from build123d import *

# Parameters (mm, degrees)
SKETCH_W        = 50
SKETCH_H        = 52
PAD_DEPTH       = 1
SKETCH001_W     = 3
SKETCH001_H     = 3
PAD001_DEPTH    = 4
FILLET_R        = 1
FILLET001_R     = 1
FILLET002_R     = 1
FILLET003_R     = 1
SKETCH002_R     = 2.75
POCKET_DEPTH    = 1
SKETCH003_W     = 2
SKETCH003_H     = 7
POCKET001_DEPTH = 1
FILLET004_R     = 0.5
SKETCH004_R     = 3.8
PAD002_DEPTH    = 2
SKETCH005_R     = 2.8
POCKET002_DEPTH = 2
SKETCH006_W     = 8
SKETCH006_H     = 36
POCKET003_DEPTH = 1
SKETCH007_W     = 6
SKETCH007_H     = 36
POCKET004_DEPTH = 1


with BuildPart() as part:
    # Sketch → Pad (new body)
    with BuildSketch(Plane.XY):
        Rectangle(SKETCH_W, SKETCH_H)
    extrude(amount=PAD_DEPTH)

    # Sketch001 (on Face6 of Pad) → Pad001 (join)
    with BuildSketch(Plane.XY.offset(1)):
        with Locations((-22.5, 23.5)):
            Rectangle(SKETCH001_W, SKETCH001_H)
        with Locations((22.5, 23.5)):
            Rectangle(SKETCH001_W, SKETCH001_H)
        with Locations((-22.5, -23.5)):
            Rectangle(SKETCH001_W, SKETCH001_H)
        with Locations((22.5, -23.5)):
            Rectangle(SKETCH001_W, SKETCH001_H)
    extrude(amount=PAD001_DEPTH)

    # Fillet
    fillet_edges = [part.edges().sort_by_distance(p)[0] for p in [
        (-25, -26, 0.5),
    ]]
    fillet(fillet_edges, radius=FILLET_R)

    # Fillet001
    fillet001_edges = [part.edges().sort_by_distance(p)[0] for p in [
        (25, -26, 0.5),
    ]]
    fillet(fillet001_edges, radius=FILLET001_R)

    # Fillet002
    fillet002_edges = [part.edges().sort_by_distance(p)[0] for p in [
        (-25, 26, 0.5),
    ]]
    fillet(fillet002_edges, radius=FILLET002_R)

    # Fillet003
    fillet003_edges = [part.edges().sort_by_distance(p)[0] for p in [
        (25, 26, 0.5),
    ]]
    fillet(fillet003_edges, radius=FILLET003_R)

    # Sketch002 (on Face1 of Fillet003) → Pocket (cut)
    with BuildSketch(Plane(origin=(0, 0, 0), x_dir=(1, 0, 0), z_dir=(0, 0, -1))):
        with Locations((-8, 20.5)):
            Circle(SKETCH002_R)
    extrude(amount=-POCKET_DEPTH, mode=Mode.SUBTRACT)

    # Sketch003 (on Face11 of Pocket) → Pocket001 (cut)
    with BuildSketch(Plane.XY.offset(1)):
        with Locations((15, -14.5)):
            Rectangle(SKETCH003_W, SKETCH003_H)
        with Locations((15, -5.5)):
            Rectangle(SKETCH003_W, SKETCH003_H)
        with Locations((11, -5.5)):
            Rectangle(SKETCH003_W, SKETCH003_H)
        with Locations((11, -14.5)):
            Rectangle(SKETCH003_W, SKETCH003_H)
        with Locations((7, -5.5)):
            Rectangle(SKETCH003_W, SKETCH003_H)
        with Locations((7, -14.5)):
            Rectangle(SKETCH003_W, SKETCH003_H)
        with Locations((3, -5.5)):
            Rectangle(SKETCH003_W, SKETCH003_H)
        with Locations((3, -14.5)):
            Rectangle(SKETCH003_W, SKETCH003_H)
    extrude(amount=-POCKET001_DEPTH, mode=Mode.SUBTRACT)

    # Fillet004
    fillet004_edges = [part.edges().sort_by_distance(p)[0] for p in [
        (0, -26, 0),
        (25, 0, 0),
        (-25, 0, 0),
        (0, 26, 0),
    ]]
    fillet(fillet004_edges, radius=FILLET004_R)

    # Sketch004 (on Face51 of Fillet004) → Pad002 (join)
    with BuildSketch(Plane.XY.offset(1)):
        with Locations((-8, -20.5)):
            Circle(SKETCH004_R)
    extrude(amount=PAD002_DEPTH)

    # Sketch005 (on Face71 of Pad002) → Pocket002 (cut)
    with BuildSketch(Plane.XY.offset(3)):
        with Locations((-8, -20.5)):
            Circle(SKETCH005_R)
    extrude(amount=-POCKET002_DEPTH, mode=Mode.SUBTRACT)

    # Sketch006 (on Face51 of Pocket002) → Pocket003 (cut)
    with BuildSketch(Plane.XY.offset(1)):
        with Locations((-21, 0)):
            Rectangle(SKETCH006_W, SKETCH006_H)
    extrude(amount=-POCKET003_DEPTH, mode=Mode.SUBTRACT)

    # Sketch007 (on Face53 of Pocket003) → Pocket004 (cut)
    with BuildSketch(Plane.XY.offset(1)):
        with Locations((22, 0)):
            Rectangle(SKETCH007_W, SKETCH007_H)
    extrude(amount=-POCKET004_DEPTH, mode=Mode.SUBTRACT)


solid = part.part
Can you work these out from the model? Positions are in its coordinate system, mm. A direction names the side the tool comes from. Coordinates: 2 decimals unless noted, no trailing zeros. Order: outer loops, then holes, each group sorted by start corner. A loop starts at its lowest first (then second) coordinate and runs counter-clockwise, first axis right, second up. Notation, with made-up numbers: M -31,4.5 L 5,4.5 A22 cw 5,32.5 Z; hole C -23.75,76.25 d7. An arc over 180 degrees is marked long. Answer as CSV lines item,"result".
(1) I'm going to push flat-ended pins straight in: pin 1 (1.5 mm diameter, centred on x = -22, z = 2.5, fed in from +Y); pin 2 (0.9 mm diameter, centred on x = -23, z = 3.5, fed in from -Y); pin 3 (6.5 mm diameter, centred on x = -8, y = -20.5, fed in from +Z). Where does each tip first touch, or does it pass through?
Geometry check:
pin 1,"y = 25"
pin 2,"y = -25"
pin 3,"z = 3"
(2) Suppose I cut it at B-B on y = -4. Please give me the cut outline in (x, z), plus the area to 3 significant figures.
Geometry check:
outline,"M -17,0 L 2,0 L 2,1 L -17,1 Z; M 4,0 L 6,0 L 6,1 L 4,1 Z; M 8,0 L 10,0 L 10,1 L 8,1 Z; M 12,0 L 14,0 L 14,1 L 12,1 Z; M 16,0 L 19,0 L 19,1 L 16,1 Z"
area,"28.0 mm^2"
(3) If we mould it in two halves opening along Y, with no side actions, what happens to faces 1 (the flat face through (21, -24, 3)), 2 (the cylindrical face through (-5.414, -21.572, 2.014)), 3 (the flat face through (22, -25, 3))? For each: released by +Y, released by -Y, zero draft, split by the parting line, or undercut.
Geometry check:
face 1,"zero draft"
face 2,"undercut"
face 3,"released by -Y"
(4) Suppose I cut it at A-A on x = -8. Please give me the cut outline in (y, z).
Geometry check:
outline,"M -26,0.5 A0.5 ccw -25.5,0 L -23.25,0 L -23.25,1 L -23.3,1 L -23.3,3 L -24.3,3 L -24.3,1 L -26,1 Z; M -17.75,0 L 25.5,0 A0.5 ccw 26,0.5 L 26,1 L -16.7,1 L -16.7,3 L -17.7,3 L -17.7,1 L -17.75,1 Z"
(5) Suppose I cut it at D-D on y = 19. Please give me the cut outline in (x, z).
Geometry check:
outline,"M -25,0.5 A0.5 ccw -24.5,0 L 24.5,0 A0.5 ccw 25,0.5 L 25,1 L -25,1 Z"
(6) On a 3-axis mill with a long thin cutter (end or side, diameter ignored), from which of +Z, -Z, +X, -X, +Y, -Y can I reach the whole of each face in a straight line? I mean faces 4 (the flat face through (-24, -24, 3)), 5 (the flat face through (22, 22, 3)), 6 (the flat face through (22, 25, 3)), 7 (the flat face through (24, -24, 3)), 8 (the flat face through (-10, -23, 3)). Say none if no direction works.
Geometry check:
face 4,"+Z, -X, +Y, -Y"
face 5,"+Z, +X, -X"
face 6,"+Z, +X, -X, +Y"
face 7,"+Z, +X, +Y, -Y"
face 8,"+Z, +Y, -Y"
(7) Suppose I cut it at C-C on y = -20.5. Please give me the cut outline in (x, z).
Geometry check:
outline,"M -25,0.5 A0.5 ccw -24.5,0 L -10.75,0 L -10.75,1 L -10.8,1 L -10.8,3 L -11.8,3 L -11.8,1 L -25,1 Z; M -5.25,0 L 24.5,0 A0.5 ccw 25,0.5 L 25,1 L -4.2,1 L -4.2,3 L -5.2,3 L -5.2,1 L -5.25,1 Z"
(8) Please list where these lines run through material, in increasing order: L1, parallel to X at y = -4, z = 0.45; L2, parallel to Y at x = -8, z = 0.4; L3, parallel to Y at x = -8, z = 1.6.
Geometry check:
L1,"-17 to 2, 4 to 6, 8 to 10, 12 to 14, 16 to 19"
L2,"-25.99 to -23.25, -17.75 to 25.99"
L3,"-24.3 to -23.3, -17.7 to -16.7"
